from build123d import *

# Parameters (mm, degrees)
BOSS_EXTRUDE1_DEPTH          = 9.525
SKETCH3_R                    = 3.2639
CUT_EXTRUDE1_DEPTH           = 60.143696832
SKETCH4_W                    = 3.8862
SKETCH4_H                    = 41.275
BOSS_EXTRUDE2_DEPTH          = 9.525
F_10_0_1935_DIAMETER_HOLE1_D = 4.9149


with BuildPart() as part:
    # Sketch2 → Boss-Extrude1 (new body)
    with BuildSketch(Plane.XY):
        Polygon((0, 0), (41.275, 0), (31.75, 9.525), (22.225, 9.525), (22.225, 19.05), (19.05, 22.225), (9.525, 22.225), (9.525, 31.75), (0, 41.275), align=None)
    extrude(amount=BOSS_EXTRUDE1_DEPTH)

    # Sketch3 → Cut-Extrude1 (cut, through all)
    with BuildSketch(Plane.XY.offset(9.525)):
        with Locations((4.445, 29.845)):
            Circle(SKETCH3_R)
        with Locations((4.445, 4.445)):
            Circle(SKETCH3_R)
    extrude(amount=-CUT_EXTRUDE1_DEPTH, mode=Mode.SUBTRACT)

    # Sketch4 → Boss-Extrude2 (add)
    with BuildSketch(Plane(origin=(0, 0, 0), x_dir=(-1, 0, 0), z_dir=(0, 0, -1))):
        with Locations((1.9431, 20.6375)):
            Rectangle(SKETCH4_W, SKETCH4_H)
    extrude(amount=-BOSS_EXTRUDE2_DEPTH)

    # #10 (0.1935) Diameter Hole1 (through all)
    with Locations(Plane(origin=(0, 22.225, 0), x_dir=(1, 0, 0), z_dir=(0, 1, 0))):
        with Locations((14.2875, -4.7625), (26.9875, -4.7625)):
            Hole(F_10_0_1935_DIAMETER_HOLE1_D / 2)


solid = part.part
Could you check a few things on this model? Use its own coordinates, in mm. A direction names the side the tool comes from. Give positions to 0.01 mm unless a question says otherwise; leave off trailing zeros. Order: outer loops, then holes, each group sorted by start corner. A loop starts at its lowest first (then second) coordinate and runs counter-clockwise, first axis right, second up.
Item 1: If we mould it in two halves opening along X, with no side actions, what happens to faces 3 (the face through (20.66, 20.615, 4.696)), 4 (the face through (-3.886, 20, 5)), 5 (the face through (9, 16, 9.525)), 6 (the face through (24.644, 4.696, 4.024))? For each: pulls with the +X half, pulls with the -X half, needs draft (parallel to the pull), parting line crosses it, or undercut.
Item 2: I'm going to push flat-ended pins straight in: pin 1 (3 mm diameter, centred on x = 27.5, z = 2.5, fed in from +Y) (3 decimals); pin 2 (2 mm diameter, centred on y = 22.5, z = 1.5, fed in from +X) (3 decimals); pin 3 (5 mm diameter, centred on y = 14.5, z = 7, fed in from +X) (3 decimals). Where does each tip first touch, or does it pass through?
Item 3: For faces 1 (the face through (29, 9.525, 7)), 2 (the face through (5.95, 26.95, 4.83)), which set-ups out of +Z, -Z, +X, -X, +Y, -Y let a thin tool reach every point of the face, with its end or its side?
Item 4: If we section it at D-D, the plane y = 18.5: Write out the boundary of the cut face in (x, z) (1 decimal).
Item 5: If we section it at B-B, the plane y = 6.5: Write out the boundary of the cut face in (x, z) (1 decimal), plus the area to 3 significant figures.
Item 6: I need wall thicknesses on line 1 (X direction, y = 6, z = 3) (3 decimals); line 2 (Y direction, x = 6.5, z = 3.5) (3 decimals); line 3 (Y direction, x = 7, z = 2.75) (3 decimals). Which ranges of each line are inside material? Lowest first, please.
Item 7: If we section it at C-C, the plane x = 26.5: Write out the boundary of the cut face in (y, z) (3 decimals), plus the area to 3 significant figures.
Item 8: If we section it at A-A, the plane z = 6: Write out the boundary of the cut face in (x, y) (3 decimals).
Values:
1. face 3: pulls with the +X half
1. face 4: pulls with the -X half
1. face 5: needs draft
1. face 6: undercut
2. pin 1: stops at y = 9.525
2. pin 2: stops at x = 19.775
2. pin 3: stops at x = 22.225
3. face 1: +Z, -Z, +X, +Y
3. face 2: +Z, -Z
4. outline: (-3.9, 0) - (22.2, 0) - (22.2, 9.5) - (-3.9, 9.5) - close; hole circle Ø4.9 at (14.3, 4.8)
5. outline: (-3.9, 0) - (1.9, 0) - (1.9, 9.5) - (-3.9, 9.5) - close; (7, 0) - (34.8, 0) - (34.8, 9.5) - (7, 9.5) - close; hole circle Ø4.9 at (14.3, 4.8); hole circle Ø4.9 at (27, 4.8)
5. area: 282 mm2
6. line 1: x = -3.886 to 1.575, 7.315 to 12.575, 16 to 25.275, 28.7 to 35.275
6. line 2: y = 0 to 1.909, 6.981 to 27.309, 32.381 to 34.775
6. line 3: y = 0 to 2.414, 6.476 to 27.814, 31.876 to 34.275
7. outline: (0, 0) - (9.525, 0) - (9.525, 2.354) - (0, 2.354) - close; (0, 7.171) - (9.525, 7.171) - (9.525, 9.525) - (0, 9.525) - close
7. area: 44.8 mm2
8. outline: (-3.886, 0) - (12.164, 0) - (12.164, 22.225) - (9.525, 22.225) - (9.525, 31.75) - (0, 41.275) - (-3.886, 41.275) - close; (16.411, 0) - (24.864, 0) - (24.864, 9.525) - (22.225, 9.525) - (22.225, 19.05) - (19.05, 22.225) - (16.411, 22.225) - close; (29.111, 0) - (41.275, 0) - (31.75, 9.525) - (29.111, 9.525) - close; hole circle Ø6.528 at (4.445, 4.445); hole circle Ø6.528 at (4.445, 29.845)
